Here's the drawing with two shaded views (mm, measured from the low corner). I have some questions. A direction names the side the tool comes from. Give positions to 0.01 mm unless a question says otherwise; leave off trailing zeros. Write each loop counter-clockwise with the first axis right and the second up, starting at its lowest first coordinate (ties: lowest second). Pieces come first, ordered by that corner, then holes. Notation, with made-up numbers: M 37.5,45 L 90.5,45 A19 cw 90.5,49 Z; hole C 49,79.5 d3. An arc over 180 degrees is marked long. Use one line per item in the form item = value.
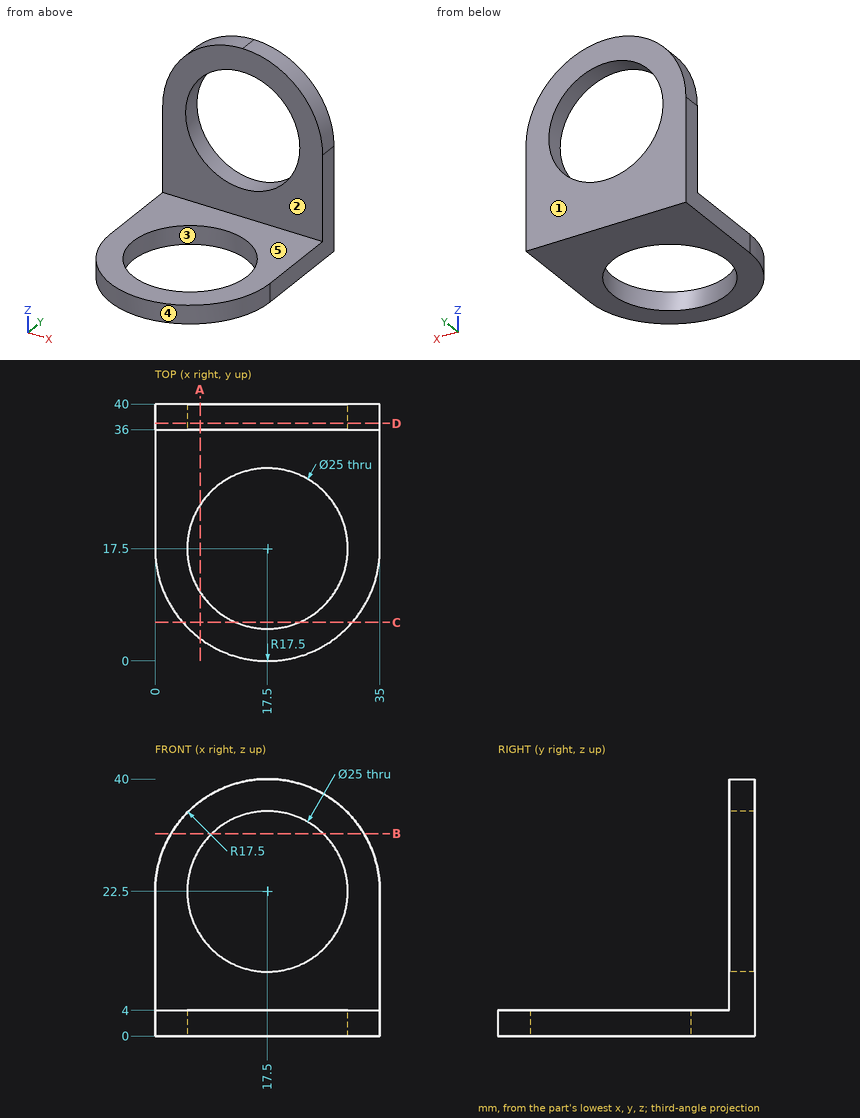
1) I want a section at A-A, the plane x = 7. Please give me the cut outline in (y, z), plus the area to 3 significant figures.
Checked values:
outline = M 3.5,0 L 10.72,0 L 10.72,4 L 3.5,4 Z; M 24.28,0 L 40,0 L 40,15.72 L 36,15.72 L 36,4 L 24.28,4 Z; M 36,29.28 L 40,29.28 L 40,36.5 L 36,36.5 Z
area = 167 mm2
2) For pin 1 Ø3 at (y, z) = (35, 29) entering from +X; pin 2 Ø8 at (x, y) = (5.5, 20.5) entering from +Z, each with a flat end and sliding along its axis, tell me the tip position at first contact or that it passes through.
Checked values:
pin_1 = 34.15
pin_2 = 4
3) If I drill on L1, parallel to Y at x = 17.5, z = 1.6; L2, parallel to Y at x = 25, z = 34.5; L3, parallel to Z at x = 27, y = 28, over which ranges is the centre line in solid material (lowest first)?
Checked values:
L1 = 0 to 5, 30 to 40
L2 = 36 to 40
L3 = 0 to 4
4) I want a section at B-B, the plane z = 31.5. Please give me the cut outline in (x, y).
Checked values:
outline = M 2.49,36 L 8.83,36 L 8.83,40 L 2.49,40 Z; M 26.17,36 L 32.51,36 L 32.51,40 L 26.17,40 Z
5) I want a section at C-C, the plane y = 6. Please give me the cut outline in (x, z).
Checked values:
outline = M 4.31,0 L 12.6,0 L 12.6,4 L 4.31,4 Z; M 22.4,0 L 30.69,0 L 30.69,4 L 22.4,4 Z
6) I want a section at D-D, the plane y = 37. Please give me the cut outline in (x, z).
Checked values:
outline = M 0,0 L 35,0 L 35,22.5 A17.5 ccw 17.5,40 A17.5 ccw 0,22.5 Z; hole C 17.5,22.5 d25
7) Thinking about a two-plate mould opening in X: for the marked faces 3, 4 and 5, which applies, released by +X, released by -X, zero draft, split by the parting line, or undercut?
Checked values:
face_3 = undercut
face_4 = split by the parting line
face_5 = zero draft
8) For the marked faces 1 and 2, which set-ups out of +Z, -Z, +X, -X, +Y, -Y let a thin tool reach every point of the face, with its end or its side?
Checked values:
face_1 = +Z, -Z, +X, -X, +Y
face_2 = +Z, +X, -X, -Y
